CAD build for the part. Positions are in the model's coordinates, mm. A direction names the side the tool comes from. Round coordinates to 2 decimals unless told otherwise and drop trailing zeros. Write each loop counter-clockwise with the first axis right and the second up, starting at its lowest first coordinate (ties: lowest second). Pieces come first, ordered by that corner, then holes. Notation, with made-up numbers: (78, -28) - (98, -28) arc R34 cw to (98, 7) - close; hole circle Ø8 at (66, 25.25). An arc over 180 degrees is marked (long way). Put each result on its own line as item: value. Start each with the question number.
Item 1: Cut at D-D (y = 17.5). Give the cut face in (x, z).
Item 2: Cut at B-B (y = 1.5). Give the cut face in (x, z).
Item 3: 3-axis set-ups, long thin cutter, end or side, ignore diameter. For faces 1 (the flat face through (17, 0, 3)), 2 (the flat face through (1, -1, 10)), 3 (the cylindrical face through (12, -12, 1)): which of +Z, -Z, +X, -X, +Y, -Y reach the whole face in a straight line?
Item 4: Cut at C-C (z = 15). Give the cut face in (x, y).
Item 5: Mould opens along X. For faces 4 (the cylindrical face through (12, 12, 1)), 5 (the flat face through (3, 0, 21)), 6 (the flat face through (0, 0, 9)), 7 (the flat face through (1, -1, 20)) say: released by +X, released by -X, zero draft, split by the parting line, or undercut.
Item 6: Cut at A-A (x = 16). Give the cut face in (y, z).
Item 7: Pin check, flat tips, straight feed: pin 1 Ø1 at (y, z) = (-18, 12.5) entering from +X; pin 2 Ø10 at (x, y) = (24, 12.5) entering from +Z; pin 3 Ø5 at (x, y) = (16, -12) entering from -Z; pin 4 Ø2.5 at (x, y) = (2, 4) entering from +Z. Stop position of each tip, or through.
Item 8: Drill centre lines: line 1 (Y direction, x = 16, z = 1.9); line 2 (Z direction, x = 19.75, y = 18). Where is each one in solid material? Low to high. Write a range as from..to.
```python
from build123d import *

# Parameters (mm, degrees)
F1_DEPTH      = 25
F1_DEPTH_BACK = 25
F2_R          = 4
F3_DEPTH      = 25
F6_DEPTH      = 25


with BuildPart() as f1:
    # F0 (on Front) → F1 (new body, two sides)
    with BuildSketch(Plane.XZ) as f1_sk:
        with BuildLine():
            Line((0, 30), (0, 0))
            Line((0, 0), (30, 0))
            ThreePointArc((30, 0), (29.12132, 2.12132), (27, 3))
            Line((27, 3), (6, 3))
            ThreePointArc((6, 3), (3.87868, 3.87868), (3, 6))
            Line((3, 6), (3, 27))
            ThreePointArc((3, 27), (2.12132, 29.12132), (0, 30))
        make_face()
    extrude(amount=F1_DEPTH)
    extrude(f1_sk.sketch, amount=-F1_DEPTH_BACK)

    # F2 (on Top) → F3 (cut)
    with BuildSketch(Plane.XY):
        with Locations((16, -12)):
            Circle(F2_R)
        with Locations((16, 12)):
            Circle(F2_R)
    extrude(amount=F3_DEPTH, mode=Mode.SUBTRACT)

    # F5 (on face) → F6 (cut)
    with BuildSketch(Plane(origin=(0, 0, 0), x_dir=(0, -1, 0), z_dir=(-1, 0, 0))):
        with BuildLine():
            ThreePointArc((-9.355084, 20), (-14.355084, 15), (-9.355084, 10))
            Line((-9.355084, 10), (10.644916, 10))
            ThreePointArc((10.644916, 10), (15.644916, 15), (10.644916, 20))
            Line((10.644916, 20), (-9.355084, 20))
        make_face()
    extrude(amount=-F6_DEPTH, mode=Mode.SUBTRACT)


solid = f1.part
```
Output values:
1. outline: (0, 0) - (30, 0) arc R3 ccw to (27, 3) - (6, 3) arc R3 cw to (3, 6) - (3, 27) arc R3 ccw to (0, 30) - close
2. outline: (0, 0) - (30, 0) arc R3 ccw to (27, 3) - (6, 3) arc R3 cw to (3, 6) - (3, 10) - (0, 10) - close; (0, 20) - (3, 20) - (3, 27) arc R3 ccw to (0, 30) - close
3. face 1: +Z, +X, +Y, -Y
3. face 2: +X, -X
3. face 3: +Z, -Z
4. outline: (0, -25) - (3, -25) - (3, -15.64) - (0, -15.64) - close; (0, 14.36) - (3, 14.36) - (3, 25) - (0, 25) - close
5. face 4: undercut
5. face 5: released by +X
5. face 6: released by -X
5. face 7: zero draft
6. outline: (-25, 0) - (-16, 0) - (-16, 3) - (-25, 3) - close; (-8, 0) - (8, 0) - (8, 3) - (-8, 3) - close; (16, 0) - (25, 0) - (25, 3) - (16, 3) - close
7. pin 1: x = 3
7. pin 2: z = 3
7. pin 3: through
7. pin 4: z = 29.9
8. line 1: -25..-16, -8..8, 16..25
8. line 2: 0..3
